Can you work these out from the drawing? Everything is in mm from the part's minimum corner. A direction names the side the tool comes from. Round coordinates to 2 decimals unless told otherwise and drop trailing zeros. Order: outer loops, then holes, each group sorted by start corner. A loop starts at its lowest first (then second) coordinate and runs counter-clockwise, first axis right, second up. Notation, with made-up numbers: (8.25, -5) -> (28.25, -5) arc R28 cw to (28.25, 34) -> close; hole circle Ø6 at (47.5, 3). An arc over 180 degrees is marked (long way). One line per item, written item: value.
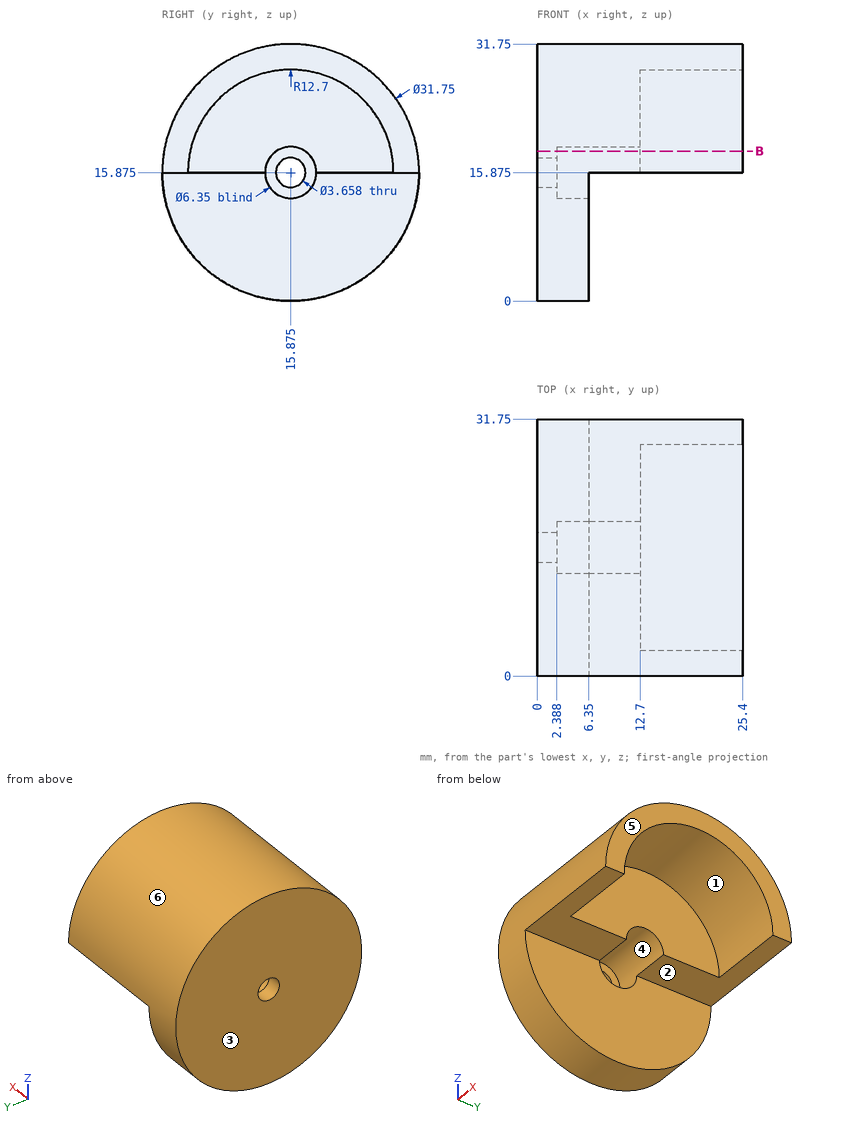
Q1. If we mould it in two halves opening along Y, with no side actions, what happens to the marked faces 4, 5 and 6? For each: pulls with the +Y half, pulls with the -Y half, needs draft (parallel to the pull), parting line crosses it, or undercut.
Answers:
face 4: undercut
face 5: needs draft
face 6: parting line crosses it
Q2. Which directions (+Z, -Z, +X, -X, +Y, -Y) give clear straight access to the entire face, cutting with the end or side of a thin tool? Please do the marked faces 1, 2 and 3.
Answers:
face 1: -Z, +X
face 2: -Z, +X, +Y, -Y
face 3: +Z, -Z, -X, +Y, -Y
Q3. For P1, Ø14, axis at x = 13, y = 7.5, coming from the -Z side (1 decimal); P2, Ø6.5, axis at x = 19.5, y = 26.5, coming from the -Z side (3 decimals); P3, Ø8, axis at y = 16, z = 6, coming from the +X side, each with a flat end and sliding along its axis, tell me the tip position at first contact or that it passes through.
Answers:
P1: z = 1.3
P2: z = 15.875
P3: x = 6.35
Q4. I want a section at B-B on z = 18.5. Write out the boundary of the cut face in (x, y).
Answers:
outline: (0, 0.22) -> (25.4, 0.22) -> (25.4, 3.45) -> (12.7, 3.45) -> (12.7, 14.09) -> (2.39, 14.09) -> (2.39, 17.66) -> (12.7, 17.66) -> (12.7, 28.3) -> (25.4, 28.3) -> (25.4, 31.53) -> (0, 31.53) -> close
Q5. I need wall thicknesses on line 1 along Y through (x, z) = (8.25, 16); line 2 along X through (y, z) = (29.5, 9); line 3 along Y through (x, z) = (17.5, 17) (1 decimal). Which ranges of each line are inside material? Lowest first, please.
Answers:
line 1: 0 to 12.7, 19.05 to 31.75
line 2: 0 to 6.35
line 3: 0 to 3.2, 28.5 to 31.7
